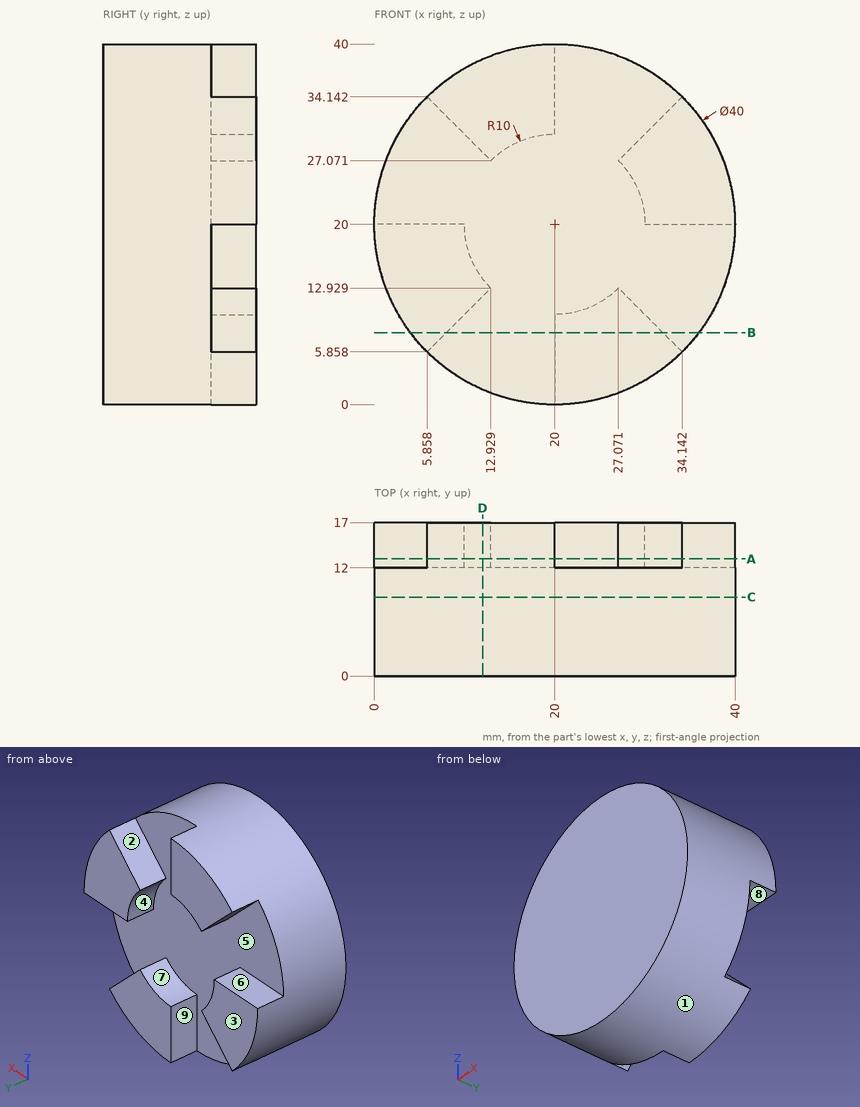
Source: three-view drawing plus pictorial views. Frame: mm from the lowest corner of the part. A direction names the side the tool comes from. Round coordinates to 2 decimals unless told otherwise and drop trailing zeros. Loops run counter-clockwise (first coordinate to the right, second up) from the corner with the lowest first, then second, coordinate; pieces in that order, holes last.
Q1. Section D-D, the plane x = 12. Return loops of the section in (y, z), plus the area to 3 significant figures.
Q2. Ray query, line 1 (Y direction, x = 32, z = 11.5); line 2 (X direction, y = 1.5, z = 20.5); line 3 (X direction, y = 15, z = 5.5) (1 decimal). Return the intervals inside material, ascending.
Q3. Access query for the marked faces 5, 6, 7, 8 and 9. Directions: +Z, -Z, +X, -X, +Y, -Y. A direction counts if a zero-diameter tool reaches every point of the face in a straight line with its end or side. Return the directions, or none.
Q4. Section C-C, the plane y = 8.75. Return loops of the section in (x, z), plus the area to 3 significant figures.
Q5. Section B-B, the plane z = 8. Return loops of the section in (x, y), plus the area to 3 significant figures.
Q6. Section A-A, the plane y = 13. Return loops of the section in (x, z), plus the area to 3 significant figures.
Q7. First-contact query: P1, Ø1.5, axis at y = 15, z = 36.5, coming from the +X side; P2, Ø2, axis at x = 17.5, y = 15, coming from the -Z side; P3, Ø1, axis at y = 12, z = 26.5, coming from the -X side. Flat tips, straight axial feed; report the tip coordinate or a pass-through.
Q8. Mould query, pull axis X, two halves, no side actions, for the marked faces 1, 2, 3 and 4. Classes: pulls with the +X half, pulls with the -X half, needs draft (parallel to the pull), parting line crosses it, or undercut.
Solutions:
1. outline: (0, 1.67) - (12, 1.67) - (12, 12) - (17, 12) - (17, 14) - (12, 14) - (12, 28) - (17, 28) - (17, 38.33) - (0, 38.33) - close
1. area: 502 mm2
2. line 1: y = 0 to 12
2. line 2: x = 0.01 to 39.99
2. line 3: x = 20 to 33.8
3. face 5: +Y
3. face 6: -X, +Y
3. face 7: +Z, +Y
3. face 8: +X, +Y
3. face 9: -Z, +Y
4. outline: circle Ø40 at (20, 20)
4. area: 1,260 mm2
5. outline: (4, 0) - (36, 0) - (36, 12) - (32, 12) - (32, 17) - (20, 17) - (20, 12) - (8, 12) - (8, 17) - (4, 17) - close
5. area: 464 mm2
6. outline: (0, 20) arc R20 ccw to (5.86, 5.86) - (12.93, 12.93) arc R10 cw to (10, 20) - close; (5.86, 34.14) - (12.93, 27.07) arc R10 cw to (20, 30) - (20, 40) arc R20 ccw to start; (20, 0) arc R20 ccw to (34.14, 5.86) - (27.07, 12.93) arc R10 cw to (20, 10) - close; (27.07, 27.07) arc R10 cw to (30, 20) - (40, 20) arc R20 ccw to (34.14, 34.14) - close
6. area: 471 mm2
7. P1: stops at x = 20
7. P2: stops at z = 29.37
7. P3: stops at x = 0.92
8. face 1: parting line crosses it
8. face 2: undercut
8. face 3: needs draft
8. face 4: pulls with the -X half
